Check sheet for the modelled part. Datum: model origin and axes. Units: mm. Face numbers are marked on the shaded views. A direction names the side the tool comes from. Coordinates: 2 decimals unless noted, no trailing zeros. Order: outer loops, then holes, each group sorted by start corner. A loop starts at its lowest first (then second) coordinate and runs counter-clockwise, first axis right, second up.
1. Cross-section at A-A (y = 2.1). Enter the section's corners in (x, z), then the cut area to 3 significant figures.
2. Gauge pin test, flat ends, axial feed: pin 1 Ø2 at (x, z) = (-15.5, 0) entering from -Y; pin 2 Ø1.5 at (x, y) = (16, 2) entering from -Z; pin 3 Ø2 at (y, z) = (1, -13.5) entering from +X; pin 4 Ø2 at (x, z) = (-16.5, -13.5) entering from +Y. Record the tip position at first contact, or that the pin passes through.
3. Draft check along X on the marked faces 1 and 2. Enter one of: released by +X, released by -X, zero draft, split by the parting line, or undercut.
4. Cross-section at B-B (x = 0). Enter the section's corners in (y, z), then the cut area to 3 significant figures.
5. Set-up check for the marked faces 3, 4 and 5: record each of +Z, -Z, +X, -X, +Y, -Y from which the full face is reachable in a straight line by a thin tool's end or side.
6. Cross-section at D-D (x = -13). Enter the section's corners in (y, z), then the cut area to 3 significant figures.
7. Cross-section at C-C (z = -16). Enter the section's corners in (x, y).
8. Thickness scan on line 1 (X direction, y = 2.3, z = -1.5); line 2 (Y direction, x = -13, z = -18); line 3 (X direction, y = 1.55, z = -10). Record the ranges inside material, lowest first.
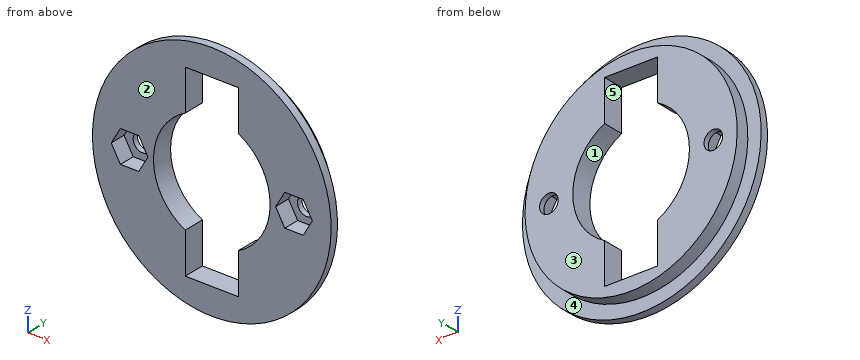
```python
from build123d import *

# Parameters (mm, degrees)
SKETCH1_R           = 22.5
BOSS_EXTRUDE2_DEPTH = 4
CUT_EXTRUDE1_START  = -2.5
SKETCH2_R           = 22.5
SKETCH2_R_2         = 20
CUT_EXTRUDE1_DEPTH  = 2.5
CUT_EXTRUDE2_DEPTH  = 33.070235422
SKETCH4_R           = 1.75
CUT_EXTRUDE3_DEPTH  = 33.070235422
CUT_EXTRUDE4_DEPTH  = 3


with BuildPart() as part:
    # Sketch1 → Boss-Extrude2 (new body)
    with BuildSketch(Plane(origin=(0, 0, 0), x_dir=(1, 0, 0), z_dir=(0, 1, 0))):
        with Locations(Location((0, 0, 0), (0, 0, 270))):
            Circle(SKETCH1_R)
    extrude(amount=BOSS_EXTRUDE2_DEPTH)

    # Sketch2 → Cut-Extrude1 (cut)
    with BuildSketch(Plane(origin=(0, 4, 0), x_dir=(1, 0, 0), z_dir=(0, 1, 0)).offset(CUT_EXTRUDE1_START)):
        with Locations(Location((0, 0, 0), (0, 0, 270))):
            Circle(SKETCH2_R)
        with Locations(Location((0, 0, 0), (0, 0, 270))):
            Circle(SKETCH2_R_2, mode=Mode.SUBTRACT)
    extrude(amount=CUT_EXTRUDE1_DEPTH, mode=Mode.SUBTRACT)

    # Sketch3 → Cut-Extrude2 (cut, through all)
    with BuildSketch(Plane(origin=(0, 4, 0), x_dir=(1, 0, 0), z_dir=(0, 1, 0))):
        with BuildLine():
            Line((5, -9.797958971), (5, -17.5))
            Line((5, -17.5), (-5, -17.5))
            Line((-5, -17.5), (-5, -9.797958971))
            ThreePointArc((-5, -9.797958971), (-11, 0), (-5, 9.797958971))
            Line((-5, 9.797958971), (-5, 17.5))
            Line((-5, 17.5), (5, 17.5))
            Line((5, 17.5), (5, 9.797958971))
            ThreePointArc((5, 9.797958971), (11, 0), (5, -9.797958971))
        make_face()
    extrude(amount=-CUT_EXTRUDE2_DEPTH, mode=Mode.SUBTRACT)

    # Sketch4 → Cut-Extrude3 (cut, through all)
    with BuildSketch(Plane(origin=(0, 4, 0), x_dir=(1, 0, 0), z_dir=(0, 1, 0))):
        with Locations(Location((15.5, 0, 0), (0, 0, 270))):
            Circle(SKETCH4_R)
        with Locations(Location((-15.5, 0, 0), (0, 0, 90))):
            Circle(SKETCH4_R)
    extrude(amount=-CUT_EXTRUDE3_DEPTH, mode=Mode.SUBTRACT)

    # Sketch5 → Cut-Extrude4 (cut)
    with BuildSketch(Plane.XZ):
        Polygon((13.767949192, -3), (12.035898385, 0), (13.767949192, 3), (17.232050808, 3), (18.964101615, 0), (17.232050808, -3), align=None)
        Polygon((-12.035898385, 0), (-13.767949192, 3), (-17.232050808, 3), (-18.964101615, 0), (-17.232050808, -3), (-13.767949192, -3), align=None)
    extrude(amount=-CUT_EXTRUDE4_DEPTH, mode=Mode.SUBTRACT)


solid = part.part
```
Data:
1. outline: circle Ø40 at (0, 0); hole (-18.96, 0) - (-17.23, -3) - (-13.77, -3) - (-12.04, 0) - (-13.77, 3) - (-17.23, 3) - close; hole (-5, -17.5) - (5, -17.5) - (5, -9.8) arc R11 ccw to (5, 9.8) - (5, 17.5) - (-5, 17.5) - (-5, 9.8) arc R11 ccw to (-5, -9.8) - close; hole (12.04, 0) - (13.77, -3) - (17.23, -3) - (18.96, 0) - (17.23, 3) - (13.77, 3) - close
1. area: 676 mm2
2. pin 1: passes through
2. pin 2: stops at z = -16.37
2. pin 3: stops at x = 18.71
2. pin 4: stops at y = 1.5
3. face 1: undercut
3. face 2: zero draft
4. outline: (0, -22.5) - (1.5, -22.5) - (1.5, -20) - (4, -20) - (4, -17.5) - (0, -17.5) - close; (0, 17.5) - (4, 17.5) - (4, 20) - (1.5, 20) - (1.5, 22.5) - (0, 22.5) - close
4. area: 27.5 mm2
5. face 3: +Z, -Z, +X, -X, +Y
5. face 4: +Y
5. face 5: +Y, -Y
6. outline: (0, -18.36) - (1.5, -18.36) - (1.5, -15.2) - (4, -15.2) - (4, 15.2) - (1.5, 15.2) - (1.5, 18.36) - (0, 18.36) - (0, 1.67) - (3, 1.67) - (3, -1.67) - (0, -1.67) - close
6. area: 121 mm2
7. outline: (-15.82, 0) - (-5, 0) - (-5, 4) - (-12, 4) - (-12, 1.5) - (-15.82, 1.5) - close; (5, 0) - (15.82, 0) - (15.82, 1.5) - (12, 1.5) - (12, 4) - (5, 4) - close
8. line 1: x = -19.94 to -18.1, -12.9 to -10.9, 10.9 to 12.9, 18.1 to 19.94
8. line 2: y = 0 to 1.5
8. line 3: x = -17.32 to -5, 5 to 17.32
